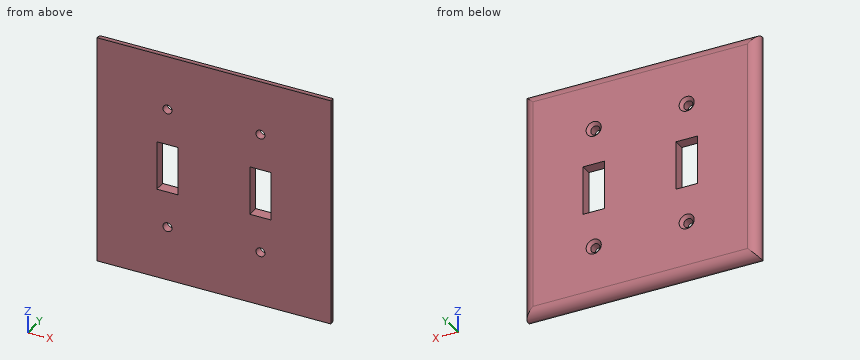
```python
from build123d import *

# Parameters (mm, degrees)
SKETCH1_W           = 116
SKETCH1_H           = 114.3
SKETCH1_R           = 2.25
SKETCH1_W_2         = 10.6
SKETCH1_H_2         = 24.3
BOSS_EXTRUDE1_DEPTH = 5.5
FILLET1_R           = 4.75
CHAMFER1_SIZE       = 1.5


with BuildPart() as part:
    # Sketch1 → Boss-Extrude1 (new body)
    with BuildSketch(Plane(origin=(0, 0, 0), x_dir=(1, 0, 0), z_dir=(0, 1, 0))):
        with Locations((-3.024594732, -5.827064496)):
            Rectangle(SKETCH1_W, SKETCH1_H)
        with Locations((-26.074594732, 24.322935504)):
            Circle(SKETCH1_R, mode=Mode.SUBTRACT)
        with Locations((-26.074594732, -35.977064496)):
            Circle(SKETCH1_R, mode=Mode.SUBTRACT)
        with Locations((20.025405268, -35.977064496)):
            Circle(SKETCH1_R, mode=Mode.SUBTRACT)
        with Locations((20.025405268, 24.322935504)):
            Circle(SKETCH1_R, mode=Mode.SUBTRACT)
        with Locations((-26.074594732, -5.827064496)):
            Rectangle(SKETCH1_W_2, SKETCH1_H_2, mode=Mode.SUBTRACT)
        with Locations((20.025405268, -5.827064496)):
            Rectangle(SKETCH1_W_2, SKETCH1_H_2, mode=Mode.SUBTRACT)
    extrude(amount=BOSS_EXTRUDE1_DEPTH)

    # Fillet1
    fillet1_edges = [part.edges().sort_by_distance(p)[0] for p in [
        (54.975405268, 5.5, 5.827064496),
        (-3.024594732, 5.5, -51.322935504),
        (-61.024594732, 5.5, 5.827064496),
        (-3.024594732, 5.5, 62.977064496),
    ]]
    fillet(fillet1_edges, radius=FILLET1_R)

    # Chamfer1
    chamfer1_edges = [part.edges().sort_by_distance(p)[0] for p in [
        (17.775405268, 5.5, 35.977064496),
        (-28.324594732, 5.5, 35.977064496),
        (-28.324594732, 5.5, -24.322935504),
        (17.775405268, 5.5, -24.322935504),
    ]]
    chamfer(chamfer1_edges, length=CHAMFER1_SIZE)


solid = part.part
```
Geometry: final body of the model. Coordinates: model frame, mm. Coordinates: 2 decimals unless noted, no trailing zeros. Write each loop counter-clockwise with the first axis right and the second up, starting at its lowest first coordinate (ties: lowest second). Pieces come first, ordered by that corner, then holes. Notation, with made-up numbers: M 43.25,87.25 L 62.25,87.25 A15 ccw 62.25,105.25 Z; hole C 54,88.25 d10. An arc over 180 degrees is marked long. Use CSV: the item, a comma, the result in double quotes. Start each with the question number.
1. Cut plane B-B on y = 2.2. Return the cut outline in (x, z).
2. Ray query, probe 1 along X at (y, z) = (0.85, 16); probe 2 along X at (y, z) = (1.05, -24); probe 3 along Z at (x, y) = (-26, 2.9). Return the intervals inside material, ascending.
3. Cut plane D-D on z = -39. Return the cut outline in (x, y), plus the area to 3 significant figures.
4. Cut plane C-C on x = 12. Return the cut outline in (y, z).
5. First-contact query: P1, Ø5, axis at x = -26.07, z = -24.32, coming from the +Y side; P2, Ø1.6, axis at x = -25.5, y = 2, coming from the +Z side; P3, Ø2, axis at x = -14.5, y = 4.5, coming from the +Z side; P4, Ø3.5, axis at x = 20.03, z = 35.98, coming from the -Y side. Flat tips, straight axial feed; report the tip coordinate or a pass-through.
6. Cut plane A-A on z = 4.5. Return the cut outline in (x, y).
Entries:
1,outline,"M -60.8,-51.1 L 54.75,-51.1 L 54.75,62.75 L -60.8,62.75 Z; hole M -31.37,-6.32 L -20.77,-6.32 L -20.77,17.98 L -31.37,17.98 Z; hole C -26.07,-24.32 d4.5; hole C -26.07,35.98 d4.5; hole M 14.73,-6.32 L 25.33,-6.32 L 25.33,17.98 L 14.73,17.98 Z; hole C 20.03,-24.32 d4.5; hole C 20.03,35.98 d4.5"
2,probe 1,"-61.02 to -31.37, -20.77 to 14.73, 25.33 to 54.97"
2,probe 2,"-61.02 to -28.3, -23.85 to 17.8, 22.25 to 54.97"
2,probe 3,"-50.81 to -26.57, -22.07 to -6.32, 17.98 to 33.73, 38.23 to 62.46"
3,outline,"M -61.02,0 L 54.98,0 L 54.98,0.75 A4.75 ccw 50.23,5.5 L -56.27,5.5 A4.75 ccw -61.02,0.75 Z"
3,area,"628 mm²"
4,outline,"M 0,-51.32 L 0.75,-51.32 A4.75 ccw 5.5,-46.57 L 5.5,58.23 A4.75 ccw 0.75,62.98 L 0,62.98 Z"
5,P1,"y = 4.26"
5,P2,"z = 62.96"
5,P3,"z = 62.1"
5,P4,"through"
6,outline,"M -61.02,0 L -31.37,0 L -31.37,5.5 L -56.27,5.5 A4.75 ccw -61.02,0.75 Z; M -20.77,0 L 14.73,0 L 14.73,5.5 L -20.77,5.5 Z; M 25.33,0 L 54.98,0 L 54.98,0.75 A4.75 ccw 50.23,5.5 L 25.33,5.5 Z"
